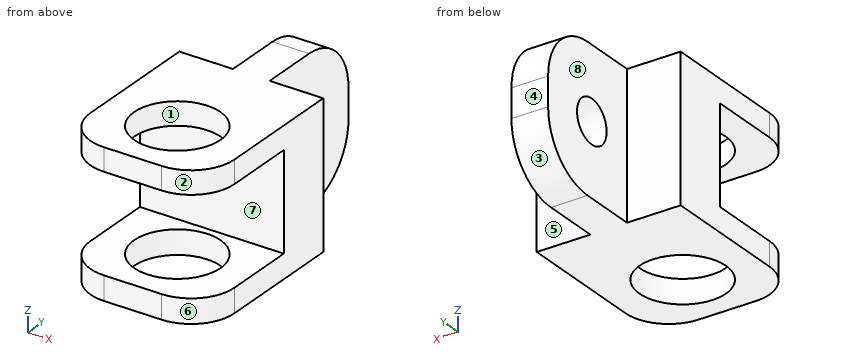
from build123d import *

# Parameters (mm, degrees)
F0_W     = 127
F0_H     = 127
F1_DEPTH = 50.8
F2_W     = 127
F2_H     = 20.286044
F2_H_2   = 21.141762
F3_DEPTH = 101.6
F5_D     = 76.2
F6_R     = 38.1
F7_W     = 32.363828
F7_H     = 127
F8_DEPTH = 101.6
F10_D    = 38.1
F11_R    = 50.8


with BuildPart() as f1:
    # F0 (on Front) → F1 (new body)
    with BuildSketch(Plane.XZ):
        Rectangle(F0_W, F0_H)
    extrude(amount=F1_DEPTH)

    # F2 (on face) → F3 (join)
    with BuildSketch(Plane.XZ.offset(50.8)):
        with Locations((0, 53.356978)):
            Rectangle(F2_W, F2_H)
        with Locations((0, -52.929119)):
            Rectangle(F2_W, F2_H_2)
    extrude(amount=F3_DEPTH)

    # F5 (through all)
    with Locations(Plane.XY.offset(63.5)):
        with Locations((0, -95.219441)):
            Hole(F5_D / 2)

    # F6
    f6_edges = [f1.edges().sort_by_distance(p)[0] for p in [
        (63.5, -152.4, 53.356978),
        (-63.5, -152.4, 53.356978),
        (63.5, -152.4, -52.929119),
        (-63.5, -152.4, -52.929119),
    ]]
    fillet(f6_edges, radius=F6_R)

    # F7 (on face) → F8 (join)
    with BuildSketch(Plane(origin=(0, 0, 0), x_dir=(-1, 0, 0), z_dir=(0, 1, 0))):
        Rectangle(F7_W, F7_H)
    extrude(amount=F8_DEPTH)

    # F10 (through all)
    with Locations(Plane(origin=(-16.181914, 0, 0), x_dir=(0, -1, 0), z_dir=(-1, 0, 0))):
        with Locations((-45.339677, 0)):
            Hole(F10_D / 2)

    # F11
    f11_edges = [f1.edges().sort_by_distance(p)[0] for p in [
        (0, 101.6, 63.5),
        (0, 101.6, -63.5),
    ]]
    fillet(f11_edges, radius=F11_R)


solid = f1.part
Verification items for the finished model (mm, model axes). Face numbers are marked on the shaded views. A direction names the side the tool comes from. Coordinates: 2 decimals unless noted, no trailing zeros. Order: outer loops, then holes, each group sorted by start corner. A loop starts at its lowest first (then second) coordinate and runs counter-clockwise, first axis right, second up. Notation, with made-up numbers: M 5,64 L 51,64 A23 ccw 51,90 Z; hole C 65.25,-20 d8. An arc over 180 degrees is marked long. One line per item, written item: value. Start each with the question number.
Item 1: Depth check by flat-ended pin: P1, Ø8, axis at y = 43, z = -15.5, coming from the +X side; P2, Ø8, axis at x = -46, z = -17.5, coming from the -Y side; P3, Ø3, axis at y = 67.5, z = 38, coming from the -X side; P4, Ø23, axis at y = 45.34, z = 0, coming from the -X side. Enter the tip coordinate at first touch or a pass-through.
Item 2: Access from +Z, -Z, +X, -X, +Y, -Y to the whole of each face (thin tool, end or side, straight path). Record for the marked faces 4, 5, 6, 7 and 8.
Item 3: Sectioned sample at B-B on z = 0. Record the cut outline in (x, y).
Item 4: Thickness scan on probe 1 along Z at (x, y) = (33, -72); probe 2 along X at (y, z) = (19, -53); probe 3 along Y at (x, z) = (0, -55). Record the ranges inside material, lowest first.
Item 5: Sectioned sample at D-D on z = -53. Record the cut outline in (x, y).
Item 6: Sectioned sample at A-A on x = -6.5. Record the cut outline in (y, z).
Item 7: Mould release check, pull along X, two halves, no side actions. Record for the marked faces 1, 2 and 3: pulls with the +X half, pulls with the -X half, needs draft (parallel to the pull), parting line crosses it, or undercut.
Item 8: Sectioned sample at C-C on y = -129.5. Record the cut outline in (x, z).
Calculated:
1. P1: x = 16.18
1. P2: y = -50.8
1. P3: x = -16.18
1. P4: through
2. face 4: +Z, -Z, +X, -X, +Y
2. face 5: +Z, -Z, +X, +Y
2. face 6: +Z, -Z, +X, -Y
2. face 7: +X, -X, -Y
2. face 8: +Z, -Z, -X, +Y
3. outline: M -63.5,-50.8 L 63.5,-50.8 L 63.5,0 L 16.18,0 L 16.18,26.29 L -16.18,26.29 L -16.18,0 L -63.5,0 Z; M -16.18,64.39 L 16.18,64.39 L 16.18,101.6 L -16.18,101.6 Z
4. probe 1: -63.5 to -42.36, 43.21 to 63.5
4. probe 2: -16.18 to 16.18
4. probe 3: -152.4 to -133.32, -57.12 to 78.93
5. outline: M -63.5,-114.3 A38.1 ccw -25.4,-152.4 L 25.4,-152.4 A38.1 ccw 63.5,-114.3 L 63.5,0 L 16.18,0 L 16.18,81.73 L -16.18,81.73 L -16.18,0 L -63.5,0 Z; hole C 0,-95.22 d76.2
6. outline: M -152.4,-63.5 L -132.76,-63.5 L -132.76,-42.36 L -152.4,-42.36 Z; M -152.4,43.21 L -132.76,43.21 L -132.76,63.5 L -152.4,63.5 Z; M -57.68,-63.5 L 50.8,-63.5 A50.8 ccw 101.6,-12.7 L 101.6,12.7 A50.8 ccw 50.8,63.5 L -57.68,63.5 L -57.68,43.21 L -50.8,43.21 L -50.8,-42.36 L -57.68,-42.36 Z; hole C 45.34,0 d38.1
7. face 1: undercut
7. face 2: pulls with the +X half
7. face 3: needs draft
8. outline: M -60.34,-63.5 L -16.63,-63.5 L -16.63,-42.36 L -60.34,-42.36 Z; M -60.34,43.21 L -16.63,43.21 L -16.63,63.5 L -60.34,63.5 Z; M 16.63,-63.5 L 60.34,-63.5 L 60.34,-42.36 L 16.63,-42.36 Z; M 16.63,43.21 L 60.34,43.21 L 60.34,63.5 L 16.63,63.5 Z
